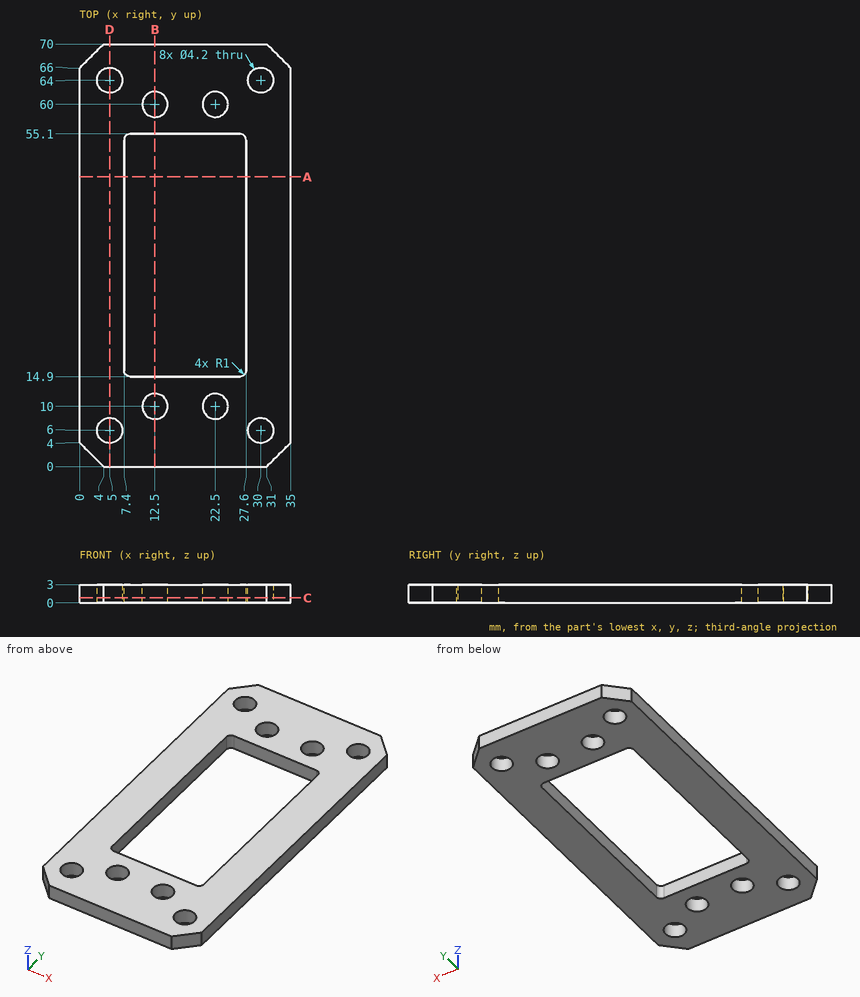
Study the drawing (mm; zero at the part's minimum x, y, z) and answer. Round coordinates to 2 decimals unless told otherwise and drop trailing zeros. Write each loop counter-clockwise with the first axis right and the second up, starting at its lowest first coordinate (ties: lowest second). Pieces come first, ordered by that corner, then holes. Notation, with made-up numbers: (88.25, 36) - (143.25, 36) arc R21 cw to (143.25, 42) - close; hole circle Ø2 at (67, -18.75). An arc over 180 degrees is marked (long way). Return JSON: item names as keys, results as strings. Group by question number.
Q1. Find the intervals of material crossed by L1, parallel to Y at x = 22.5, z = 1.1; L2, parallel to Y at x = 30, z = 1.1; L3, parallel to X at y = 64, z = 2.4, in increasing order.
Q2. The part is cut by section D-D on x = 5. Write down the section's boundary in (y, z), then the cut area to 3 significant figures.
Q3. This flat-tipped pin is pushed along its axis until it touches: pin 1 Ø2.5 at (x, y) = (12.5, 10) entering from +Z. Where does it stop, or does it pass through?
Q4. The part is cut by section A-A on y = 48. Write down the section's boundary in (x, z).
Q5. The part is cut by section C-C on z = 0.8. Count the separate pieces of the cut face and the enclosed holes in it, then the cut area to 3 significant figures.
Q6. The part is cut by section B-B on x = 12.5. Write down the section's boundary in (y, z).
Solved:
{
 "1": {"L1": "0 to 7.9, 12.1 to 14.9, 55.1 to 57.9, 62.1 to 70", "L2": "0 to 3.9, 8.1 to 61.9, 66.1 to 70", "L3": "0 to 2.9, 7.1 to 27.9, 32.1 to 35"},
 "2": {"outline": "(0, 0) - (3.9, 0) - (3.9, 3) - (0, 3) - close; (8.1, 0) - (61.9, 0) - (61.9, 3) - (8.1, 3) - close; (66.1, 0) - (70, 0) - (70, 3) - (66.1, 3) - close", "area": "185 mm²"},
 "3": {"pin 1": "through"},
 "4": {"outline": "(0, 0) - (7.4, 0) - (7.4, 3) - (0, 3) - close; (27.6, 0) - (35, 0) - (35, 3) - (27.6, 3) - close"},
 "5": {"separate pieces": "1", "enclosed holes": "9", "area": "1,500 mm²"},
 "6": {"outline": "(0, 0) - (7.9, 0) - (7.9, 3) - (0, 3) - close; (12.1, 0) - (14.9, 0) - (14.9, 3) - (12.1, 3) - close; (55.1, 0) - (57.9, 0) - (57.9, 3) - (55.1, 3) - close; (62.1, 0) - (70, 0) - (70, 3) - (62.1, 3) - close"}
}
